Build history of the part. All positions in model axes, mm. A direction names the side the tool comes from. Give positions to 0.01 mm unless a question says otherwise; leave off trailing zeros. Order: outer loops, then holes, each group sorted by start corner. A loop starts at its lowest first (then second) coordinate and runs counter-clockwise, first axis right, second up. Notation, with made-up numbers: M 20.5,-7.5 L 62.5,-7.5 A9 cw 62.5,4.5 Z; hole C -28.5,-4 d11. An arc over 180 degrees is marked long. One line per item, written item: value.
from build123d import *

# Parameters (mm, degrees)
EXTRUDE_THIN3_DEPTH      = 664
EXTRUDE_THIN3_DEPTH_BACK = 818
SKETCH1_W                = 25.4
SKETCH1_H                = 30.226
CUT_EXTRUDE1_DEPTH       = 674
CUT_EXTRUDE1_DEPTH_BACK  = 743
SKETCH4_W                = 80
SKETCH4_H                = 25.4
BOSS_EXTRUDE1_DEPTH      = 3.048
CUT_EXTRUDE2_DEPTH       = 178


with BuildPart() as part:
    # Sketch1 → Extrude-Thin3 (new, two sides: drawn at the far end of the back side and taken through both)
    with BuildSketch(Plane(origin=(0, 0, 0), x_dir=(0, 0, -1), z_dir=(1, 0, 0)).offset(-EXTRUDE_THIN3_DEPTH_BACK)):
        with Locations((-93.98, -189.611)):
            Rectangle(SKETCH1_W, SKETCH1_H)
    extrude(amount=EXTRUDE_THIN3_DEPTH + EXTRUDE_THIN3_DEPTH_BACK)

    # Sketch3 → Cut-Extrude1 (cut, two sides: drawn at the far end of the back side and taken through both)
    with BuildSketch(Plane(origin=(0, 0, 0), x_dir=(0, 0, -1), z_dir=(1, 0, 0)).offset(-CUT_EXTRUDE1_DEPTH_BACK)):
        with BuildLine():
            Line((-81.650098629, -187.772933629), (-84.268930353, -202.625066371))
            ThreePointArc((-84.268930353, -202.625066371), (-85.137661517, -204.129752886), (-86.770342046, -204.724))
            Line((-86.770342046, -204.724), (-101.189657954, -204.724))
            ThreePointArc((-101.189657954, -204.724), (-102.822338483, -204.129752886), (-103.691069647, -202.625066371))
            Line((-103.691069647, -202.625066371), (-106.309901371, -187.772933629))
            Line((-106.309901371, -187.772933629), (-112.090636736, -187.772933629))
            Line((-112.090636736, -187.772933629), (-112.090636736, -212.168156894))
            Line((-112.090636736, -212.168156894), (-76.546243061, -212.168156894))
            Line((-76.546243061, -212.168156894), (-76.546243061, -187.772933629))
            Line((-76.546243061, -187.772933629), (-81.650098629, -187.772933629))
        make_face()
    extrude(amount=CUT_EXTRUDE1_DEPTH + CUT_EXTRUDE1_DEPTH_BACK, mode=Mode.SUBTRACT)


with BuildPart() as body_2:
    # Mirror3: mirrored copy
    add(part.part.mirror(Plane.ZX.offset(-206.248)))


with BuildPart() as part_1:
    add(part.part)

    add(body_2.part)  # Boss-Extrude1 merges body 2
    # Sketch4 → Boss-Extrude1 (add)
    with BuildSketch(Plane(origin=(0, -207.772, 0), x_dir=(1, 0, 0), z_dir=(0, 1, 0))):
        with Locations((-778, -93.98)):
            Rectangle(SKETCH4_W, SKETCH4_H)
    extrude(amount=BOSS_EXTRUDE1_DEPTH)

    # Sketch6 → Cut-Extrude2 (cut)
    with BuildSketch(Plane.XY):
        Polygon((-638.463603746, -185.674), (-742.95, -185.674), (-744.293611593, -193.294), (-746.309028982, -204.724), (-742.95, -208.788), (-740.934582611, -220.218), (-739.590971018, -227.838), (-638.640030294, -227.838), (-621.247897552, -210.445867257), (-621.247897552, -202.889706194), align=None)
    extrude(amount=CUT_EXTRUDE2_DEPTH, mode=Mode.SUBTRACT)


solid = part_1.part
1) Saw through at A-A, the plane x = -543. Write the cut outline in (y, z), then the cut area to 3 significant figures.
Check values:
outline: M -238,81.28 L -224.72,81.28 L -224.72,81.65 L -209.87,84.27 A2.54 ccw -207.77,86.77 L -207.77,101.19 A2.54 ccw -209.87,103.69 L -224.72,106.31 L -224.72,106.68 L -238,106.68 Z; M -204.72,86.77 A2.54 ccw -202.63,84.27 L -187.77,81.65 L -187.77,81.28 L -174.5,81.28 L -174.5,106.68 L -187.77,106.68 L -187.77,106.31 L -202.63,103.69 A2.54 ccw -204.72,101.19 Z
area: 1,410 mm^2
2) Pin check, flat tip, straight feed: pin 1 (10 mm diameter, centred on x = 158.5, y = -219.5, fed in from -Z). Stop position of the tip, or through.
Check values:
pin 1: z = 81.69
3) Tool access for faces 1 (the face through (-87, -186, 106.68)), 2 (the face through (-690, -185.674, 94)): list every direction of +Z, -Z, +X, -X, +Y, -Y with a clear straight run to the whole face (end or side of a thin tool).
Check values:
face 1: +Z, +X, -X, +Y, -Y
face 2: +Z, -Z
4) Drill centre lines: probe 1 along X at (y, z) = (-225, 102); probe 2 along Y at (x, z) = (-121.5, 91); probe 3 along Y at (x, z) = (-640, 101.5). Where is each one in solid material? Low to high. Write a range as from..to.
Check values:
probe 1: -818..-740.09, -635.8..664
probe 2: -238..-207.77, -204.72..-174.5
probe 3: -238..-227.84, -185.67..-174.5
5) Mould opens along Y. For faces 3 (the face through (-87, -174.498, 94)), 4 (the face through (-818, -207, 94)), 5 (the face through (-690, -227.838, 94)) say: released by +Y, released by -Y, zero draft, split by the parting line, or undercut.
Check values:
face 3: released by +Y
face 4: zero draft
face 5: undercut
